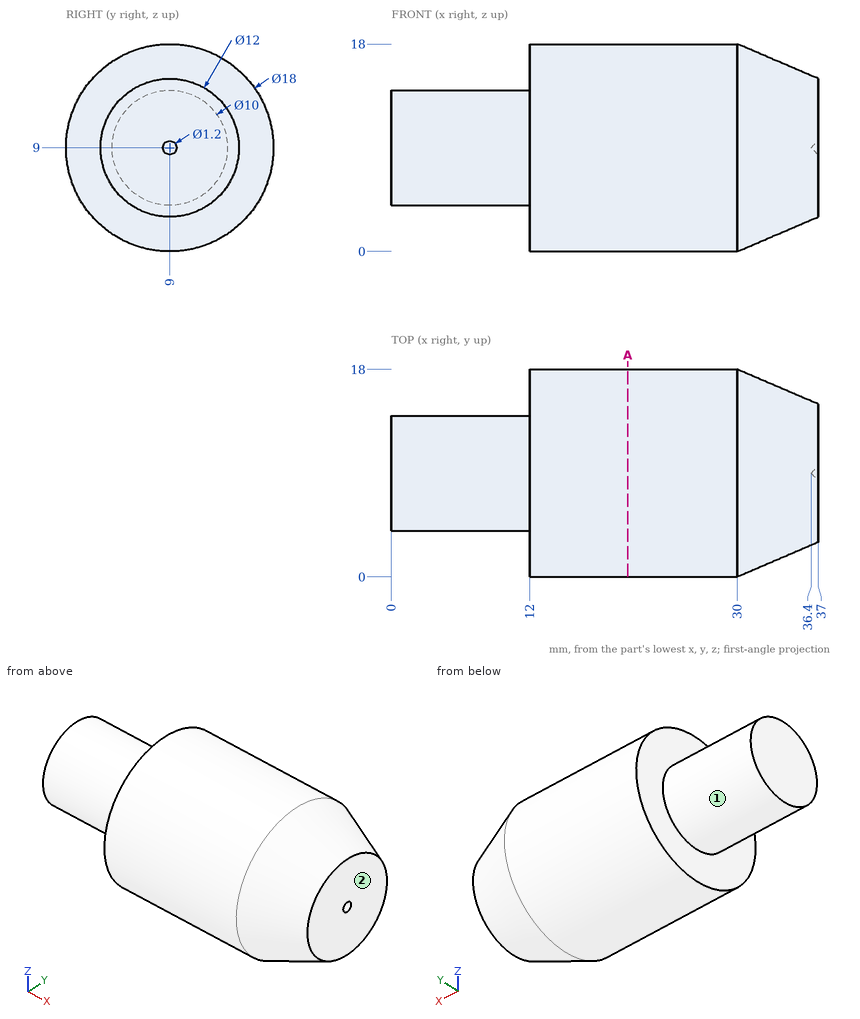
Check sheet for the drawn part. Datum: minimum x, y, z corner. Units: mm. A direction names the side the tool comes from. Give positions to 0.01 mm unless a question says otherwise; leave off trailing zeros. Write each loop counter-clockwise with the first axis right and the second up, starting at its lowest first coordinate (ties: lowest second). Pieces come first, ordered by that corner, then holes. Notation, with made-up numbers: M 84.5,32.25 L 127.5,32.25 A25 ccw 127.5,63.25 Z; hole C -36,85.25 d3. An arc over 180 degrees is marked long. One line per question, with ' | ' between items.
1) Section check A-A on x = 20.5. Enter the section's corners in (y, z).
Result:
outline: C 9,9 d18
2) Thickness scan on line 1 along Y through (x, z) = (17.5, 9.25); line 2 along Z through (x, y) = (34.5, 14); line 3 along X through (y, z) = (4.75, 4.75). Record the ranges inside material, lowest first. Write a range as [from, to].
Result:
line 1: y = [0, 18] | line 2: z = [4, 14] | line 3: x = [12, 36.98]
3) Set-up check for the marked faces 1 and 2: record each of +Z, -Z, +X, -X, +Y, -Y from which the full face is reachable in a straight line by a thin tool's end or side.
Result:
face 1: -X | face 2: +Z, -Z, +X, +Y, -Y
4) Gauge pin test, flat ends, axial feed: pin 1 Ø1 at (x, y) = (18, 3.5) entering from -Z; pin 2 Ø3 at (x, y) = (12.5, 14) entering from -Z; pin 3 Ø4 at (x, y) = (6.5, 8) entering from +Z. Record the tip position at first contact, or that the pin passes through.
Result:
pin 1: stops at z = 1.52 | pin 2: stops at z = 0.71 | pin 3: stops at z = 14
